Input: part model. Units: mm. Frame: model coordinates. A direction names the side the tool comes from. Coordinates: 2 decimals unless noted, no trailing zeros. Loops run counter-clockwise (first coordinate to the right, second up) from the corner with the lowest first, then second, coordinate; pieces in that order, holes last. Notation, with made-up numbers: (-31, 19.25) -> (-17, 19.25) arc R15 cw to (-17, 46.25) -> close; hole circle Ø3 at (75.25, 63.5). An arc over 180 degrees is marked (long way). Put each result on its own line as item: value. Start each with the question number.
1) Cut plane A-A (x = 50). Return the cut outline in (y, z).
2) Pull-direction query (X, two-part tool) for faces 5 (the flat face through (57.4, -3, -3)), 6 (the cylindrical face through (73.56, 7.09, 0.93)), 7 (the flat face through (80, -5.3, -2.1)), 8 (the flat face through (0, 0, 0)); classes: pulls with the +X half, pulls with the -X half, needs draft (parallel to the pull), parting line crosses it, or undercut.
3) Cut plane B-B (x = 75). Return the cut outline in (y, z).
4) Contact query for flat-ended pins moving along their axis: P1, Ø3, axis at x = 20, z = 3.5, coming from the +Y side; P2, Ø3, axis at x = 60, y = -1, coming from the +Z side; P3, Ø1, axis at x = 23.5, z = 6.5, coming from the -Y side. Output: stop coordinate, or through.
5) Set-up query: faces 1 (the cylindrical face through (107.865, -3.905, 0.867)), 2 (the flat face through (31.4, 7, 0)), 3 (the flat face through (110.4, 0, 0)), 4 (the cylindrical face through (14.297, 3.955, -5.158)). Return all of +Z, -Z, +X, -X, +Y, -Y with unobstructed straight access to the full face (end or side cutting, diameter ignored); none if empty.
6) Material intervals for L1, parallel to X at y = 6.5, z = -2.25; L2, parallel to X at y = -3.5, z = 5; L3, parallel to X at y = 2, z = -4.25, sorted ascending.
from build123d import *

# Parameters (mm, degrees)
SKETCH_1_R       = 6.5
EXTRUDE_1_DEPTH  = 29
SKETCH_2_R       = 8
EXTRUDE_2_DEPTH  = 2.4
SKETCH_3_R       = 6.5
EXTRUDE_3_DEPTH  = 1.6
SKETCH_4_R       = 8
EXTRUDE_4_DEPTH  = 2.4
SKETCH_5_R       = 4
EXTRUDE_5_DEPTH  = 22
SKETCH_6_R       = 7.15
EXTRUDE_6_DEPTH  = 8.8
SKETCH_7_R       = 5.55
EXTRUDE_7_DEPTH  = 1.1
SKETCH_8_R       = 7.15
EXTRUDE_8_DEPTH  = 12.7
SKETCH_9_R       = 5.55
EXTRUDE_9_DEPTH  = 25.4
SKETCH_10_R      = 4
EXTRUDE_10_DEPTH = 5


with BuildPart() as part:
    # Эскиз1 → Бобышка-Вытянуть1 (new body)
    with BuildSketch(Plane(origin=(0, 0, 0), x_dir=(0, 0, -1), z_dir=(1, 0, 0))):
        with Locations(Location((0, 0, 0), (0, 0, 180))):
            Circle(SKETCH_1_R)
    extrude(amount=EXTRUDE_1_DEPTH)

    # Эскиз2 → Бобышка-Вытянуть2 (add)
    with BuildSketch(Plane(origin=(29, 0, 0), x_dir=(0, 0, -1), z_dir=(1, 0, 0))):
        Circle(SKETCH_2_R)
    extrude(amount=EXTRUDE_2_DEPTH)

    # Эскиз3 → Бобышка-Вытянуть3 (add)
    with BuildSketch(Plane(origin=(31.4, 0, 0), x_dir=(0, 0, -1), z_dir=(1, 0, 0))):
        with Locations(Location((0, 0, 0), (0, 0, 180))):
            Circle(SKETCH_3_R)
    extrude(amount=EXTRUDE_3_DEPTH)

    # Эскиз4 → Бобышка-Вытянуть4 (add)
    with BuildSketch(Plane(origin=(33, 0, 0), x_dir=(0, 0, -1), z_dir=(1, 0, 0))):
        Circle(SKETCH_4_R)
    extrude(amount=EXTRUDE_4_DEPTH)

    # Эскиз5 → Бобышка-Вытянуть5 (add)
    with BuildSketch(Plane(origin=(35.4, 0, 0), x_dir=(0, 0, -1), z_dir=(1, 0, 0))):
        Circle(SKETCH_5_R)
    extrude(amount=EXTRUDE_5_DEPTH)

    # Эскиз6 → Бобышка-Вытянуть6 (add)
    with BuildSketch(Plane(origin=(57.4, 0, 0), x_dir=(0, 0, -1), z_dir=(1, 0, 0))):
        Circle(SKETCH_6_R)
    extrude(amount=EXTRUDE_6_DEPTH)

    # Эскиз7 → Бобышка-Вытянуть7 (add)
    with BuildSketch(Plane(origin=(66.2, 0, 0), x_dir=(0, 0, -1), z_dir=(1, 0, 0))):
        Circle(SKETCH_7_R)
    extrude(amount=EXTRUDE_7_DEPTH)

    # Эскиз8 → Бобышка-Вытянуть8 (add)
    with BuildSketch(Plane(origin=(67.3, 0, 0), x_dir=(0, 0, -1), z_dir=(1, 0, 0))):
        Circle(SKETCH_8_R)
    extrude(amount=EXTRUDE_8_DEPTH)

    # Эскиз9 → Бобышка-Вытянуть9 (add)
    with BuildSketch(Plane(origin=(80, 0, 0), x_dir=(0, 0, -1), z_dir=(1, 0, 0))):
        Circle(SKETCH_9_R)
    extrude(amount=EXTRUDE_9_DEPTH)

    # Эскиз10 → Бобышка-Вытянуть10 (add)
    with BuildSketch(Plane(origin=(105.4, 0, 0), x_dir=(0, 0, -1), z_dir=(1, 0, 0))):
        Circle(SKETCH_10_R)
    extrude(amount=EXTRUDE_10_DEPTH)


solid = part.part
Results found:
1. outline: circle Ø8 at (0, 0)
2. face 5: undercut
2. face 6: needs draft
2. face 7: pulls with the +X half
2. face 8: pulls with the -X half
3. outline: circle Ø14.3 at (0, 0)
4. P1: stops at y = 6.18
4. P2: stops at z = 7.15
4. P3: stops at y = -2.5
5. face 1: +X
5. face 2: none
5. face 3: +Z, -Z, +X, +Y, -Y
5. face 4: -X
6. L1: x = 29 to 31.4, 33 to 35.4, 57.4 to 66.2, 67.3 to 80
6. L2: x = 0 to 35.4, 57.4 to 66.2, 67.3 to 80
6. L3: x = 0 to 35.4, 57.4 to 105.4
